Part print with two shaded views. Sizes in mm from the minimum x, y, z corner. A direction names the side the tool comes from. Give positions to 0.01 mm unless a question says otherwise; leave off trailing zeros. Order: outer loops, then holes, each group sorted by start corner. A loop starts at its lowest first (then second) coordinate and runs counter-clockwise, first axis right, second up. Notation, with made-up numbers: M 2,-33 L 25,-33 A15 ccw 25,-21 Z; hole C 51.25,19.25 d1. An arc over 180 degrees is marked long. Answer as CSV lines item,"result".
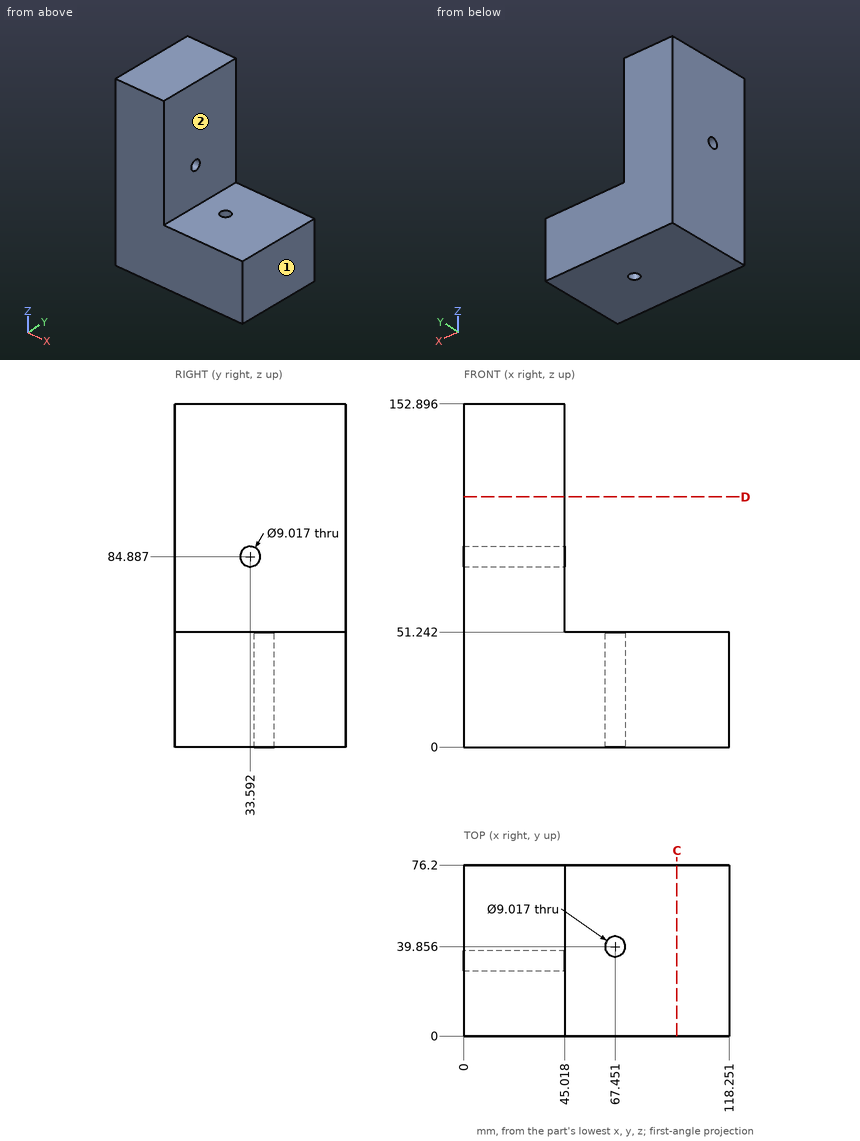
Item 1: Band-saw the part on C-C (x = 95). Give the cut face in (y, z), and give its area (3 significant figures).
Geometry says:
outline,"M 0,0 L 76.2,0 L 76.2,51.24 L 0,51.24 Z"
area,"3,900 mm2"
Item 2: Probe line 1 along Z through (x, y) = (78.5, 32); line 2 along X through (y, z) = (29.5, 146.5); line 3 along Z through (x, y) = (10, 32.5) (1 decimal). List the from-to ranges inside material, lowest first. Write a range as from..to.
Geometry says:
line 1,"z = 0..51.24"
line 2,"x = 0..45.02"
line 3,"z = 0..80.5, 89.3..152.9"
Item 3: Drop flat-ended pins along their axis: pin 1 (10.5 mm diameter, centred on x = 67.45, y = 39.86, fed in from +Z); pin 2 (10 mm diameter, centred on x = 52.5, z = 56.5, fed in from +Y). Give the stop position or say it passes through.
Geometry says:
pin 1,"stops at z = 51.24"
pin 2,"passes through"
Item 4: 3-axis set-ups, long thin cutter, end or side, ignore diameter. For the marked faces 1 and 2: which of +Z, -Z, +X, -X, +Y, -Y reach the whole face in a straight line?
Geometry says:
face 1,"+Z, -Z, +X, +Y, -Y"
face 2,"+Z, +X, +Y, -Y"
Item 5: Band-saw the part on D-D (z = 111.5). Give the cut face in (x, y), and give its area (3 significant figures).
Geometry says:
outline,"M 0,0 L 45.02,0 L 45.02,76.2 L 0,76.2 Z"
area,"3,430 mm2"
